Geometry: see drawing. Coordinates: mm, zero at the bounding-box minimum. Give positions to 0.01 mm unless a question says otherwise; leave off trailing zeros. Write each loop counter-clockwise with the first axis right and the second up, starting at its lowest first coordinate (ties: lowest second). Pieces come first, ordered by that corner, then holes. Notation, with made-up numbers: M 13,82.25 L 43,82.25 A34 cw 43,120.25 Z; hole C 49.5,39.5 d10. An arc over 180 degrees is marked long. Use a Markdown table: item, result. Add a question column.
(1) Cut plane B-B (z = 116.5). Output: boundary loops of the cut face in (x, y).
(2) Cut plane A-A (z = 17.5). Output: boundary loops of the cut face in (x, y).
(3) Pin query (flat end, axial travel): pin 1 Ø3 at (x, z) = (9, 124) entering from -Y; pin 2 Ø10 at (x, z) = (8, 144) entering from -Y; pin 3 Ø2 at (y, z) = (26, 159) entering from +X. Return the tip coordinate at first contact, or that it passes through.
(4) Material intervals for L1, parallel to X at y = 18, z = 158.5; L2, parallel to Y at x = 30, z = 149 (1 decimal); L3, parallel to X at y = 28, z = 178.5 (1 decimal), sorted ascending.
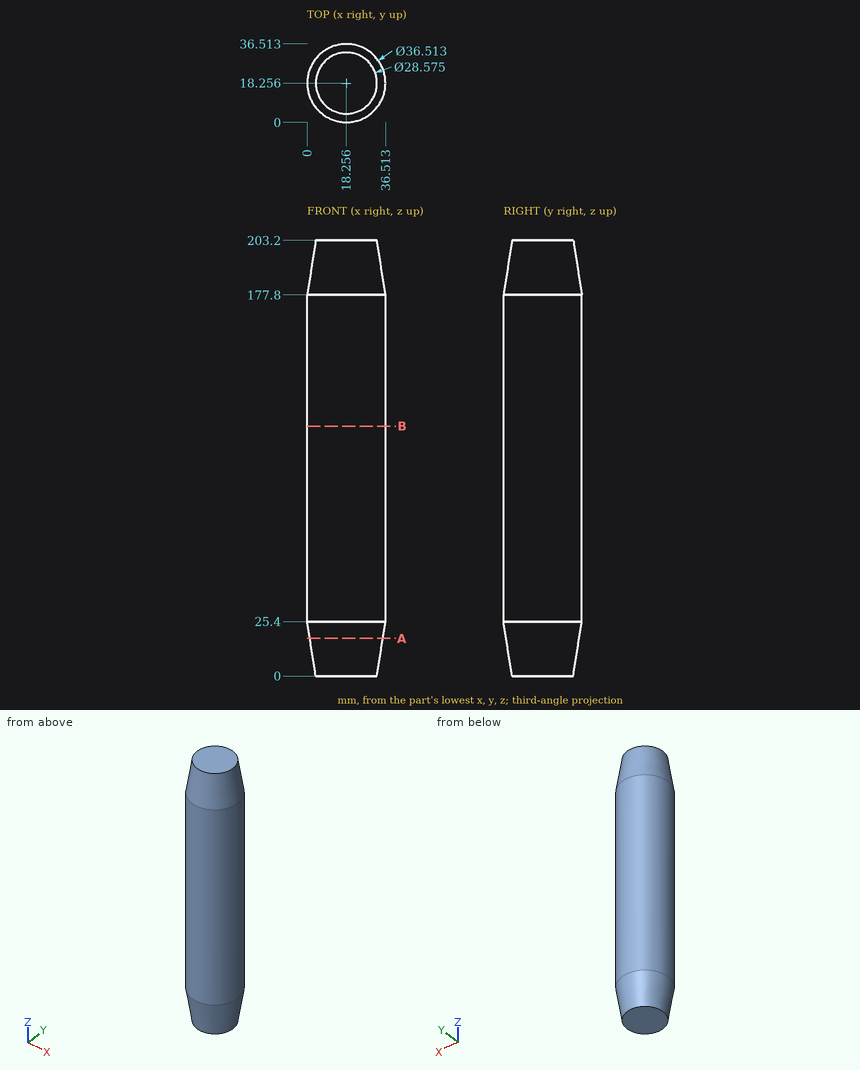
Answer list:
| question | item | result |
|---|---|---|
| 1 | outline | C 18.26,18.26 d36.51 |
| 2 | outline | C 18.26,18.26 d34.04 |
| 3 | pin 1 | y = 1.73 |
| 3 | pin 2 | y = 0.77 |
| 3 | pin 3 | x = 35.22 |
| 4 | L1 | 0 to 36.51 |
| 4 | L2 | 4.3 to 32.2 |
| 4 | L3 | 2.9 to 33.6 |
